Part model, mm, in its own coordinate system. Face numbers are marked on the shaded views. A direction names the side the tool comes from. Round coordinates to 2 decimals unless told otherwise and drop trailing zeros. Write each loop counter-clockwise with the first axis right and the second up, starting at its lowest first coordinate (ties: lowest second). Pieces come first, ordered by that corner, then holes.
1) Saw through at B-B on x = 0. Write the cut outline in (y, z).
2) Pull direction X, two halves, no side cores. Call the marked faces 1 and 2: +X half, -X half, draft (parallel to the pull), parting line (faces both ways), or undercut.
3) Saw through at A-A on x = 8.5. Write the cut outline in (y, z), and give its area (3 significant figures).
4) Drill centre lines: L1, parallel to Y at x = 8.5, z = -0.7; L2, parallel to X at y = 8.75, z = -0.9; L3, parallel to Y at x = -7.25, z = -1.1. Where is each one in solid material? Low to high.
5) Saw through at C-C on y = -8.75. Write the cut outline in (x, z).
6) Saw through at D-D on z = -2. Write the cut outline in (x, y), and give its area (3 significant figures).
7) Which spindle directions (+Z, -Z, +X, -X, +Y, -Y) get a long thin tool onto all of the face, cutting with end or side? Do the marked faces 3, 4, 5 and 6. Say none if no direction does.
8) Flat gauge pins, fed straight in: pin 1 (0.9 mm diameter, centred on x = 7, z = -1.5, fed in from -Y); pin 2 (0.9 mm diameter, centred on x = -8, z = -1, fed in from +Y); pin 3 (1.5 mm diameter, centred on y = -18, z = -2, fed in from -X). Where does each tip first touch, or does it go through?
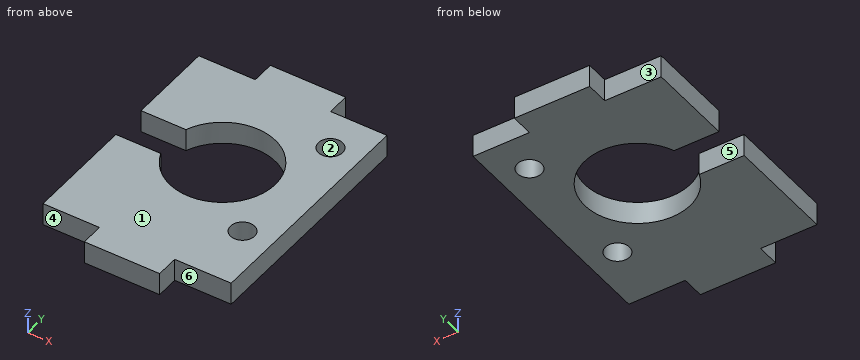
```python
from build123d import *

# Parameters (mm, degrees)
SKETCH1_R           = 1.6
BOSS_EXTRUDE1_DEPTH = 3


with BuildPart() as part:
    # Sketch1 → Boss-Extrude1 (new body)
    with BuildSketch(Plane(origin=(0, 0, 0), x_dir=(1, 0, 0), z_dir=(0, 0, -1))):
        with BuildLine():
            Line((-5, 17), (-5, 20))
            Line((-5, 20), (5, 20))
            Line((5, 20), (5, 17))
            Line((5, 17), (12.5, 17))
            Line((12.5, 17), (12.5, -14))
            Line((12.5, -14), (5, -14))
            Line((5, -14), (5, -17))
            Line((5, -17), (-5, -17))
            Line((-5, -17), (-5, -14))
            Line((-5, -14), (-12.5, -14))
            Line((-12.5, -14), (-12.5, -2.5))
            Line((-12.5, -2.5), (-6.538348415, -2.5))
            ThreePointArc((-6.538348415, -2.5), (7, 0), (-6.538348415, 2.5))
            Line((-6.538348415, 2.5), (-12.5, 2.5))
            Line((-12.5, 2.5), (-12.5, 17))
            Line((-12.5, 17), (-5, 17))
        make_face()
        with Locations(Location((8.5, 8.75, 0), (0, 0, 180))):
            Circle(SKETCH1_R, mode=Mode.SUBTRACT)
        with Locations((8.5, -8.75)):
            Circle(SKETCH1_R, mode=Mode.SUBTRACT)
    extrude(amount=BOSS_EXTRUDE1_DEPTH)


solid = part.part
```
Completed:
1. outline: (-20, -3) - (-7, -3) - (-7, 0) - (-20, 0) - close; (7, -3) - (17, -3) - (17, 0) - (7, 0) - close
2. face 1: draft
2. face 2: undercut
3. outline: (-17, -3) - (-10.35, -3) - (-10.35, 0) - (-17, 0) - close; (-7.15, -3) - (7.15, -3) - (7.15, 0) - (-7.15, 0) - close; (10.35, -3) - (14, -3) - (14, 0) - (10.35, 0) - close
3. area: 73.8 mm2
4. L1: y = -17 to -10.35, -7.15 to 7.15, 10.35 to 14
4. L2: x = -12.5 to 6.9, 10.1 to 12.5
4. L3: y = -17 to -2.5, 2.5 to 14
5. outline: (-12.5, -3) - (6.9, -3) - (6.9, 0) - (-12.5, 0) - close; (10.1, -3) - (12.5, -3) - (12.5, 0) - (10.1, 0) - close
6. outline: (-12.5, -17) - (-5, -17) - (-5, -20) - (5, -20) - (5, -17) - (12.5, -17) - (12.5, 14) - (5, 14) - (5, 17) - (-5, 17) - (-5, 14) - (-12.5, 14) - (-12.5, 2.5) - (-6.54, 2.5) arc R7 cw (long way) to (-6.54, -2.5) - (-12.5, -2.5) - close; hole circle Ø3.2 at (8.5, -8.75); hole circle Ø3.2 at (8.5, 8.75)
6. area: 637 mm2
7. face 3: +Z, -Z, -X, +Y
7. face 4: +Z, -Z, -X, -Y
7. face 5: +Z, -Z, -X
7. face 6: +Z, -Z, +X, -Y
8. pin 1: stops at y = -17
8. pin 2: stops at y = 14
8. pin 3: stops at x = -5
